from build123d import *

# Parameters (mm, degrees)
F0_W     = 44.45
F0_H     = 88.9
F1_DEPTH = 6.35
F2_W     = 6.35
F2_H     = 6.35
F2_W_2   = 12.7
F3_DEPTH = 6.35
F4_R     = 10.668
F4_W     = 27.94
F4_H     = 48.26
F4_R_2   = 1.27
F5_DEPTH = 25.4
F6_W     = 12.361424
F6_H     = 8.128
F7_DEPTH = 25.4


with BuildPart() as f1:
    # F0 (on Right) → F1 (new body)
    with BuildSketch(Plane.YZ):
        with Locations((22.225, 44.45)):
            Rectangle(F0_W, F0_H)
    extrude(amount=F1_DEPTH)

    # F2 (on face) → F3 (join)
    with BuildSketch(Plane.YZ.offset(6.35)):
        with Locations((3.175, 92.075)):
            Rectangle(F2_W, F2_H)
        with Locations((3.175, -3.175)):
            Rectangle(F2_W, F2_H)
        with Locations((41.275, 92.075)):
            Rectangle(F2_W, F2_H)
        with Locations((41.275, -3.175)):
            Rectangle(F2_W, F2_H)
        with Locations((22.225, 92.075)):
            Rectangle(F2_W_2, F2_H)
        with Locations((22.225, -3.175)):
            Rectangle(F2_W_2, F2_H)
    extrude(amount=-F3_DEPTH)

    # F4 (on face) → F5 (cut)
    with BuildSketch(Plane.YZ.offset(6.35)):
        with Locations((22.225, 13.97)):
            Circle(F4_R)
        with Locations((22.225, 59.69)):
            Rectangle(F4_W, F4_H)
        with Locations((22.225, 87.63)):
            Circle(F4_R_2)
        with Locations((22.225, 31.75)):
            Circle(F4_R_2)
    extrude(amount=-F5_DEPTH, mode=Mode.SUBTRACT)

    # F6 (on face) → F7 (cut)
    with BuildSketch(Plane.YZ.offset(6.35)):
        with Locations((6.180712, 13.97)):
            Rectangle(F6_W, F6_H)
    extrude(amount=-F7_DEPTH, mode=Mode.SUBTRACT)


solid = f1.part
Design review of the part built by this model. Coordinates are the model's own, in mm. A direction names the side the tool comes from. Coordinates: 2 decimals unless noted, no trailing zeros. Loops run counter-clockwise (first coordinate to the right, second up) from the corner with the lowest first, then second, coordinate; pieces in that order, holes last. Notation, with made-up numbers: (50.5, 45) -> (65.5, 45) arc R19 ccw to (65.5, 73) -> close; hole circle Ø5 at (-28, 52.25). An arc over 180 degrees is marked (long way). Use a Markdown table: item, result. Add a question column.
Item 1: We need section A-A, the plane y = 10.5. Write out the cut boundary in (x, z).
Item 2: Machinability: for faces 1 (the flat face through (3, 11, 0)), 2 (the flat face through (3, 28.575, 92)), 3 (the flat face through (3, 22, 35.56)), 4 (the flat face through (3, 22, 95.25)), which of the approach directions +Z, -Z, +X, -X, +Y, -Y give a long, thin tool a straight path to every point of the face, cutting with its end or side? Answer none if there is none.
Item 3: Wall thickness on L1, parallel to Y at x = 1.75, z = 65 (3 decimals); L2, parallel to Z at x = 2, y = 33; L3, parallel to Z at x = 2.75, y = 12: over which ranges is each line inside the solid? List them lowest first. Write a range as from..to.
Item 4: The part is to be moulded in two halves that separate along Y. For faces 5 (the flat face through (3, 11, 88.9)), 6 (the flat face through (3, 44.45, 44)), 7 (the flat face through (3, 0, 56)), 8 (the flat face through (3, 15.875, 92)), say which applies: +Y half, -Y half, draft (parallel to the pull), parting line (faces both ways), or undercut.
Item 5: We need section B-B, the plane z = 49. Write out the cut boundary in (x, y) (3 decimals).
Item 6: We need section C-C, the plane x = 3.25. Count the separate pieces of the cut face and the enclosed holes in it, and give its area (3 significant figures).
Item 7: We need section D-D, the plane z = 31.75. Write out the cut boundary in (x, y) (3 decimals).
Numbers:
| question | item | result |
|---|---|---|
| 1 | outline | (0, 0) -> (6.35, 0) -> (6.35, 9.91) -> (0, 9.91) -> close; (0, 18.03) -> (6.35, 18.03) -> (6.35, 35.56) -> (0, 35.56) -> close; (0, 83.82) -> (6.35, 83.82) -> (6.35, 88.9) -> (0, 88.9) -> close |
| 2 | face 1 | -Z, +X, -X |
| 2 | face 2 | +Z, +X, -X |
| 2 | face 3 | +X, -X |
| 2 | face 4 | +Z, +X, -X, +Y, -Y |
| 3 | L1 | y = 0..8.255, 36.195..44.45 |
| 3 | L2 | z = 0..35.56, 83.82..88.9 |
| 3 | L3 | z = 0..9.91, 18.03..35.56, 83.82..88.9 |
| 4 | face 5 | undercut |
| 4 | face 6 | +Y half |
| 4 | face 7 | -Y half |
| 4 | face 8 | undercut |
| 5 | outline | (0, 0) -> (6.35, 0) -> (6.35, 8.255) -> (0, 8.255) -> close; (0, 36.195) -> (6.35, 36.195) -> (6.35, 44.45) -> (0, 44.45) -> close |
| 6 | separate pieces | 1 |
| 6 | enclosed holes | 3 |
| 6 | area | 2,460 mm^2 |
| 7 | outline | (0, 0) -> (6.35, 0) -> (6.35, 20.955) -> (0, 20.955) -> close; (0, 23.495) -> (6.35, 23.495) -> (6.35, 44.45) -> (0, 44.45) -> close |
